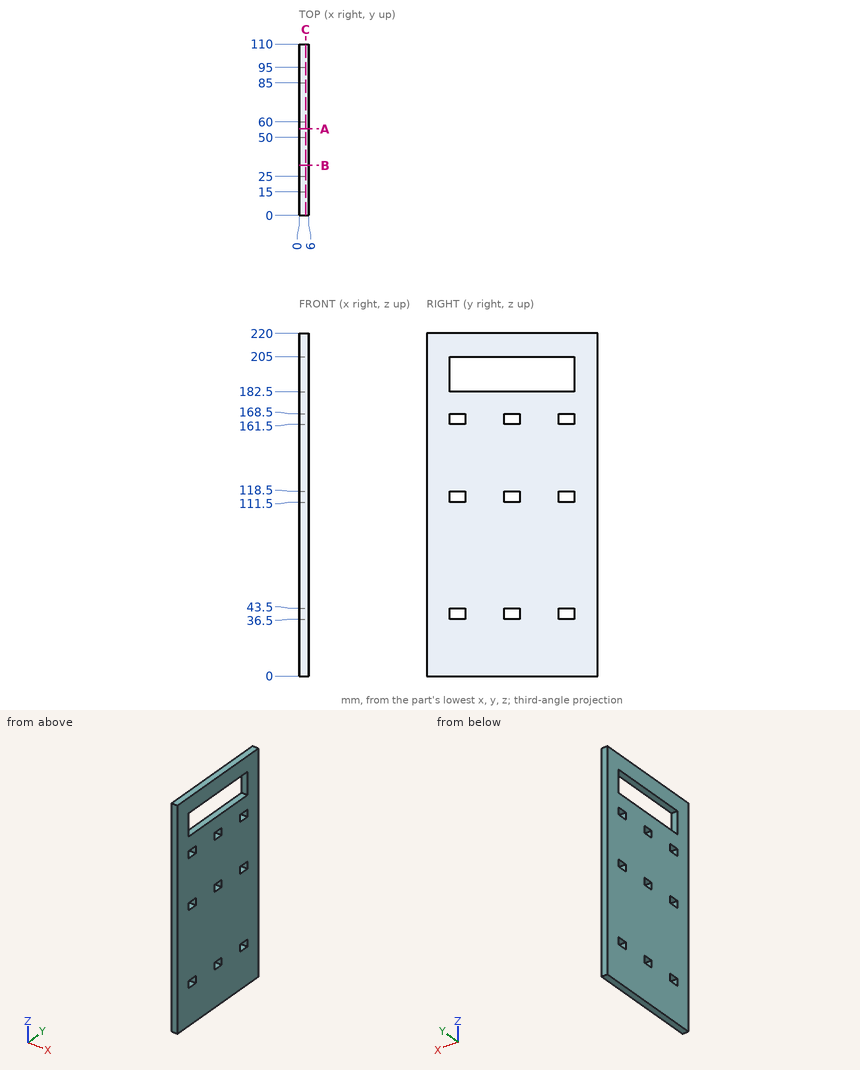
The figure shows three views and two pictorial views of one solid part (mm, origin at its lowest corner). Answer the questions. Round coordinates to 2 decimals unless told otherwise and drop trailing zeros. Write each loop counter-clockwise with the first axis right and the second up, starting at its lowest first coordinate (ties: lowest second). Pieces come first, ordered by that corner, then holes. Notation, with made-up numbers: (17, -10.75) - (21, -10.75) arc R28 ccw to (21, 9.25) - close; hole circle Ø9 at (-17.75, -20.75). An arc over 180 degrees is marked (long way). Use one line per item in the form item = value. Start each with the question number.
Item 1: A cutting plane is placed at B-B (y = 32). Write down the section's boundary in (x, z), plus the area to 4 significant figures.
Item 2: Find the intervals of material crossed by line 1 (Z direction, x = 2.8, y = 59); line 2 (Z direction, x = 3.05, y = 82); line 3 (Y direction, x = 3.55, z = 187), in increasing order. Write a range as [from, to].
Item 3: A cutting plane is placed at A-A (y = 55.5). Write down the section's boundary in (x, z).
Item 4: A cutting plane is placed at C-C (x = 4.2). Give the number of separate pieces and of enclosed holes in the cut face, plus the area to 3 significant figures.
Item 5: A flat-ended cylindrical pin translates along its axis: pin 1 Ø8 at (y, z) = (40, 149) entering from -X. Find the tip coordinate at first contact, or state that the pin passes through.
The answers:
q1.outline = (0, 0) - (6, 0) - (6, 182.5) - (0, 182.5) - close; (0, 205) - (6, 205) - (6, 220) - (0, 220) - close
q1.area = 1,185 mm^2
q2.line_1 = [0, 36.5], [43.5, 111.5], [118.5, 161.5], [168.5, 182.5], [205, 220]
q2.line_2 = [0, 182.5], [205, 220]
q2.line_3 = [0, 15], [95, 110]
q3.outline = (0, 0) - (6, 0) - (6, 36.5) - (0, 36.5) - close; (0, 43.5) - (6, 43.5) - (6, 111.5) - (0, 111.5) - close; (0, 118.5) - (6, 118.5) - (6, 161.5) - (0, 161.5) - close; (0, 168.5) - (6, 168.5) - (6, 182.5) - (0, 182.5) - close; (0, 205) - (6, 205) - (6, 220) - (0, 220) - close
q4.separate_pieces = 1
q4.enclosed_holes = 10
q4.area = 21,800 mm^2
q5.pin_1 = 0
